from build123d import *

# Parameters (mm, degrees)
EXTRUDE1_DEPTH = 150


with BuildPart() as part:
    # Sketch2 → Extrude1 (new body)
    with BuildSketch(Plane.XY):
        with BuildLine():
            Line((18.5, -5.8), (18.5, -5))
            Line((18.5, -5), (14, -5))
            Line((14, -5), (14, -10.05))
            Line((14, -10.05), (11.464213562, -10.05))
            Line((11.464213562, -10.05), (7.5, -6.085786438))
            Line((7.5, -6.085786438), (7.5, 6.085786438))
            Line((7.5, 6.085786438), (11.464213562, 10.05))
            Line((11.464213562, 10.05), (14, 10.05))
            Line((14, 10.05), (14, 5))
            Line((14, 5), (18.5, 5))
            Line((18.5, 5), (18.5, 5.8))
            Line((18.5, 5.8), (20, 5.8))
            Line((20, 5.8), (20, 17.369192104))
            ThreePointArc((20, 17.369192104), (19.229454207, 19.229454207), (17.369192104, 20))
            Line((17.369192104, 20), (13.3, 20))
            ThreePointArc((13.3, 20), (-10.246655814, 10.246655814), (-20, -13.3))
            Line((-20, -13.3), (-20, -17.369192104))
            ThreePointArc((-20, -17.369192104), (-19.229454207, -19.229454207), (-17.369192104, -20))
            Line((-17.369192104, -20), (-5.8, -20))
            Line((-5.8, -20), (-5.8, -18.5))
            Line((-5.8, -18.5), (-5, -18.5))
            Line((-5, -18.5), (-5, -14))
            Line((-5, -14), (-10.05, -14))
            Line((-10.05, -14), (-10.05, -11.464213562))
            Line((-10.05, -11.464213562), (-6.085786438, -7.5))
            Line((-6.085786438, -7.5), (6.085786438, -7.5))
            Line((6.085786438, -7.5), (10.05, -11.464213562))
            Line((10.05, -11.464213562), (10.05, -14))
            Line((10.05, -14), (5, -14))
            Line((5, -14), (5, -18.5))
            Line((5, -18.5), (5.8, -18.5))
            Line((5.8, -18.5), (5.8, -20))
            Line((5.8, -20), (17.369192104, -20))
            ThreePointArc((17.369192104, -20), (19.229454207, -19.229454207), (20, -17.369192104))
            Line((20, -17.369192104), (20, -5.8))
            Line((20, -5.8), (18.5, -5.8))
        make_face()
        with BuildLine():
            Line((2.397915762, 5.5), (1.998263135, 4.583333333))
            ThreePointArc((1.998263135, 4.583333333), (0, 5), (-1.998263135, 4.583333333))
            Line((-1.998263135, 4.583333333), (-2.397915762, 5.5))
            Line((-2.397915762, 5.5), (-5.5, 5.5))
            Line((-5.5, 5.5), (-5.5, 2.397915762))
            Line((-5.5, 2.397915762), (-4.583333333, 1.998263135))
            ThreePointArc((-4.583333333, 1.998263135), (-5, 0), (-4.583333333, -1.998263135))
            Line((-4.583333333, -1.998263135), (-5.5, -2.397915762))
            Line((-5.5, -2.397915762), (-5.5, -5.5))
            Line((-5.5, -5.5), (-2.397915762, -5.5))
            Line((-2.397915762, -5.5), (-1.998263135, -4.583333333))
            ThreePointArc((-1.998263135, -4.583333333), (0, -5), (1.998263135, -4.583333333))
            Line((1.998263135, -4.583333333), (2.397915762, -5.5))
            Line((2.397915762, -5.5), (5.5, -5.5))
            Line((5.5, -5.5), (5.5, -2.397915762))
            Line((5.5, -2.397915762), (4.583333333, -1.998263135))
            ThreePointArc((4.583333333, -1.998263135), (5, 0), (4.583333333, 1.998263135))
            Line((4.583333333, 1.998263135), (5.5, 2.397915762))
            Line((5.5, 2.397915762), (5.5, 5.5))
            Line((5.5, 5.5), (2.397915762, 5.5))
        make_face(mode=Mode.SUBTRACT)
        with BuildLine():
            Line((9.438262309, 10.852475871), (6.585786438, 8))
            Line((6.585786438, 8), (-6.585786438, 8))
            Line((-6.585786438, 8), (-8.467768079, 9.881981642))
            ThreePointArc((-8.467768079, 9.881981642), (1.586686602, 16.264138568), (13.28390541, 18.499995927))
            Line((13.28390541, 18.499995927), (14.5, 18.500611416))
            Line((14.5, 18.500611416), (14.5, 17.25))
            ThreePointArc((14.5, 17.25), (16.444543648, 16.444543648), (17.25, 14.5))
            Line((17.25, 14.5), (18.5, 14.5))
            Line((18.5, 14.5), (18.5, 9.5))
            ThreePointArc((18.5, 9.5), (17, 8), (15.5, 9.5))
            Line((15.5, 9.5), (15.5, 11.288691855))
            ThreePointArc((15.5, 11.288691855), (15.325221818, 11.668469118), (14.923076923, 11.782739262))
            ThreePointArc((14.923076923, 11.782739262), (12.555456352, 12.555456352), (11.782739262, 14.923076923))
            ThreePointArc((11.782739262, 14.923076923), (11.668469118, 15.325221818), (11.288691855, 15.5))
            Line((11.288691855, 15.5), (10.438262309, 15.5))
            ThreePointArc((10.438262309, 15.5), (9.731155527, 15.207106781), (9.438262309, 14.5))
            Line((9.438262309, 14.5), (9.438262309, 10.852475871))
        make_face(mode=Mode.SUBTRACT)
        with BuildLine():
            Line((11.75, -15.5), (11.75, -14.5))
            ThreePointArc((11.75, -14.5), (12.555456352, -12.555456352), (14.5, -11.75))
            Line((14.5, -11.75), (15.5, -11.75))
            Line((15.5, -11.75), (15.5, -9.5))
            ThreePointArc((15.5, -9.5), (17, -8), (18.5, -9.5))
            Line((18.5, -9.5), (18.5, -14.5))
            Line((18.5, -14.5), (17.25, -14.5))
            ThreePointArc((17.25, -14.5), (16.444543648, -16.444543648), (14.5, -17.25))
            Line((14.5, -17.25), (14.5, -18.5))
            Line((14.5, -18.5), (9.5, -18.5))
            ThreePointArc((9.5, -18.5), (8, -17), (9.5, -15.5))
            Line((9.5, -15.5), (11.75, -15.5))
        make_face(mode=Mode.SUBTRACT)
        with BuildLine():
            Line((-18.500611416, -14.5), (-18.499995927, -13.28390541))
            ThreePointArc((-18.499995927, -13.28390541), (-16.264138568, -1.586686602), (-9.881981642, 8.467768079))
            Line((-9.881981642, 8.467768079), (-8, 6.585786438))
            Line((-8, 6.585786438), (-8, -6.585786438))
            Line((-8, -6.585786438), (-10.852475871, -9.438262309))
            Line((-10.852475871, -9.438262309), (-14.5, -9.438262309))
            ThreePointArc((-14.5, -9.438262309), (-15.207106781, -9.731155527), (-15.5, -10.438262309))
            Line((-15.5, -10.438262309), (-15.5, -11.288691855))
            ThreePointArc((-15.5, -11.288691855), (-15.325221818, -11.668469118), (-14.923076923, -11.782739262))
            ThreePointArc((-14.923076923, -11.782739262), (-12.555456352, -12.555456352), (-11.782739262, -14.923076923))
            ThreePointArc((-11.782739262, -14.923076923), (-11.668469118, -15.325221818), (-11.288691855, -15.5))
            Line((-11.288691855, -15.5), (-9.5, -15.5))
            ThreePointArc((-9.5, -15.5), (-8, -17), (-9.5, -18.5))
            Line((-9.5, -18.5), (-14.5, -18.5))
            Line((-14.5, -18.5), (-14.5, -17.25))
            ThreePointArc((-14.5, -17.25), (-16.444543648, -16.444543648), (-17.25, -14.5))
            Line((-17.25, -14.5), (-18.500611416, -14.5))
        make_face(mode=Mode.SUBTRACT)
    extrude(amount=-EXTRUDE1_DEPTH)


solid = part.part
Work out the finished part from the listing and answer in its coordinate system (mm). A direction names the side the tool comes from. Give positions to 0.01 mm unless a question says otherwise; leave off trailing zeros. Return JSON: item names as keys, results as strings.
Q1. Find the intervals of material crossed by line 1 along X through (y, z) = (4, -129.5); line 2 along Y through (x, z) = (-11, -22); line 3 along X through (y, z) = (-12, -83), in increasing order. Write a range as [from, to].
Answer below:
{"line 1": "x = [-15.15, -13.38], [-8, -5.5], [5.5, 7.5]", "line 2": "y = [-20, -18.5], [-15.5, -9.44], [7.21, 9.47]", "line 3": "x = [-19.97, -18.47], [-13.35, -10.05], [10.05, 13.35], [18.5, 20]"}
Q2. The mould has two halves that part along X. Classify faces 4 (the face through (20, 12, -74)), 5 (the face through (14, 8, -74)), 6 (the face through (4, -5.5, -74)), 7 (the face through (12, -20, -74)): pulls with the +X half, pulls with the -X half, needs draft (parallel to the pull), parting line crosses it, or undercut.
Answer below:
{"face 4": "pulls with the +X half", "face 5": "undercut", "face 6": "undercut", "face 7": "needs draft"}
Q3. Each of these flat-tipped pins is pushed along its axis until it touches: pin 1 (5.5 mm diameter, centred on x = -12, z = -59.5, fed in from +Y); pin 2 (1.6 mm diameter, centred on x = 19.5, z = -53, fed in from -Y); pin 3 (1.5 mm diameter, centred on y = -11, z = -51, fed in from -X). Where does it stop, or does it pass through?
Answer below:
{"pin 1": "stops at y = 11.2", "pin 2": "stops at y = -19.64", "pin 3": "stops at x = -19.96"}
Q4. Find section A-A, the plane z = -82. State how many separate pieces and enclosed holes the cut face has, and give its area (3 significant figures).
Answer below:
{"separate pieces": "1", "enclosed holes": "4", "area": "489 mm^2"}
Q5. Which of the six approach directions +Z, -Z, +X, -X, +Y, -Y give full straight-line access (tool end or side, diameter ignored) to faces 1 (the face through (16, 5, -74)), 2 (the face through (-5, -16, -74)), 3 (the face through (18.5, 12, -74))?
Answer below:
{"face 1": "+Z, -Z, +X", "face 2": "+Z, -Z, -Y", "face 3": "+Z, -Z"}
